Source: CAD feature listing. Evaluate the final solid. Frame: model axes, mm. Face numbers are marked on the shaded views. Give positions to 0.01 mm unless a question says otherwise; leave off trailing zeros. Loops run counter-clockwise (first coordinate to the right, second up) from the corner with the lowest first, then second, coordinate; pieces in that order, holes last. Notation, with made-up numbers: (55.5, 57.5) - (71.5, 57.5) arc R15 cw to (71.5, 74.5) - close; hole circle Ø8 at (-4.5, -6). An arc over 180 degrees is marked (long way). Put each result on its own line as item: value.
```python
from build123d import *

# Parameters (mm, degrees)
SKETCH1_R           = 4.993252943
BOSS_EXTRUDE2_DEPTH = 5


with BuildPart() as part:
    # Sketch1 → Boss-Extrude2 (new, symmetric)
    with BuildSketch(Plane.XY):
        with BuildLine():
            Line((299.568188368, 38.981558344), (319.568188368, 38.981558344))
            ThreePointArc((319.568188368, 38.981558344), (334.568188368, 23.981558344), (319.568188368, 8.981558344))
            Line((319.568188368, 8.981558344), (299.568188368, 8.981558344))
            Line((299.568188368, 8.981558344), (299.568188368, 38.981558344))
        make_face()
        with Locations((319.568188368, 23.981558344)):
            Circle(SKETCH1_R, mode=Mode.SUBTRACT)
    extrude(amount=BOSS_EXTRUDE2_DEPTH, both=True)

    # Sketch3 → Revolve3 (revolve)
    with BuildSketch(Plane.XY, mode=Mode.PRIVATE) as revolve3_sk:
        Polygon((291.998587327, 45.654710618), (291.998587327, 47.281219247), (299.568188368, 47.281219247), (299.568188368, 38.981558344), (299.568188368, 23.981558344), (286.998587327, 23.981558344), (286.998587327, 39.61078701), (36.998587327, 39.61078701), (36.998587327, 45.654710618), align=None)
    revolve(revolve3_sk.sketch.rotate(Axis((286.998587327, 23.981558344, 0), (1, 0, 0)), 90), axis=Axis((286.998587327, 23.981558344, 0), (1, 0, 0)))


solid = part.part
```
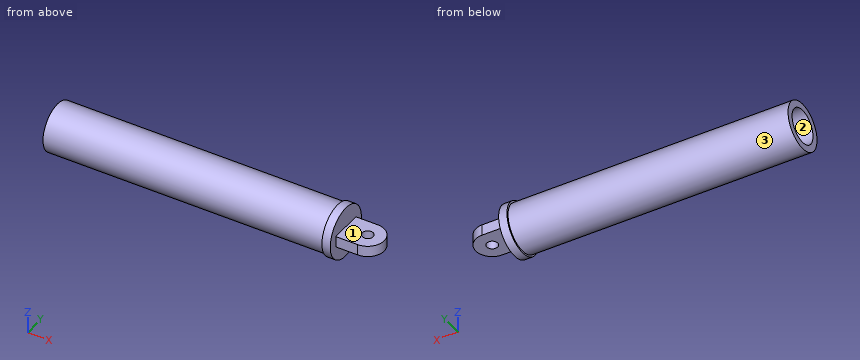
1) Section query C-C, the plane x = 79. Output: boundary loops of the cut face in (y, z).
Check result:
outline: circle Ø43.35 at (23.98, 0); hole circle Ø31.26 at (23.98, 0)
2) Section query D-D, the plane z = 12. Output: boundary loops of the cut face in (x, y), plus the area to 3 significant figures.
Check result:
outline: (37, 5.93) - (292, 5.93) - (292, 4.01) - (299.57, 4.01) - (299.57, 43.95) - (292, 43.95) - (292, 42.03) - (37, 42.03) - (37, 34) - (287, 34) - (287, 13.97) - (37, 13.97) - close
area: 4,500 mm²
3) Section query B-B, the plane y = 12.5. Output: boundary loops of the cut face in (x, z).
Check result:
outline: (37, -18.38) - (292, -18.38) - (292, -20.27) - (299.57, -20.27) - (299.57, -5) - (329.22, -5) - (329.22, 5) - (299.57, 5) - (299.57, 20.27) - (292, 20.27) - (292, 18.38) - (37, 18.38) - (37, 10.6) - (287, 10.6) - (287, -10.6) - (37, -10.6) - close
4) Pin query (flat end, axial travel): P1, Ø12, axis at x = 91, y = 40, coming from the -Z side; P2, Ø4, axis at x = 117, z = 2, coming from the +Y side; P3, Ø9, axis at x = 316.5, y = 31, coming from the +Z side. Return the tip coordinate at first contact, or that it passes through.
Check result:
P1: z = -19.22
P2: y = 45.65
P3: z = 5
5) Material intervals for line 1 along X through (y, z) = (24.5, -4); line 2 along Y through (x, z) = (104, 0); line 3 along Y through (x, z) = (253, 1), sorted ascending. Write a range as [from, to].
Check result:
line 1: [287, 314.6], [324.53, 334.56]
line 2: [2.31, 8.35], [39.61, 45.65]
line 3: [2.33, 8.38], [39.58, 45.63]
6) Section query A-A, the plane z = 0. Output: boundary loops of the cut face in (x, y), plus the area to 3 significant figures.
Check result:
outline: (37, 2.31) - (292, 2.31) - (292, 0.68) - (299.57, 0.68) - (299.57, 8.98) - (319.57, 8.98) arc R15 ccw to (319.57, 38.98) - (299.57, 38.98) - (299.57, 47.28) - (292, 47.28) - (292, 45.65) - (37, 45.65) - (37, 39.61) - (287, 39.61) - (287, 8.35) - (37, 8.35) - close; hole circle Ø9.99 at (319.57, 23.98)
area: 4,470 mm²
7) Mould query, pull axis Z, two halves, no side actions, for the marked faces 1, 2 and 3. Classes: pulls with the +Z half, pulls with the -Z half, needs draft (parallel to the pull), parting line crosses it, or undercut.
Check result:
face 1: pulls with the +Z half
face 2: undercut
face 3: parting line crosses it
